from build123d import *

# Parameters (mm, degrees)
F1_DEPTH = 25
F2_R     = 1.2
F3_T     = -2.5
F4_DEPTH = 25
F6_DEPTH = 3
F7_SIZE  = 1.2


with BuildPart() as f1:
    # F0 (on Top) → F1 (new body)
    with BuildSketch(Plane.XY):
        with BuildLine():
            Line((0, -23.9775525033), (0, 0))
            Line((0, 0), (0, 26.0224474967))
            add(Edge.make_bspline(
                [(0, 26.0224474967), (-17.6971325381, 20.4363816506), (-33.2169395037, 16.3747998881), (-39.9791178567, 18.1051199008)],
                knots=[0, 0, 0, 0, 0.723504363, 0.723504363, 0.723504363, 0.723504363], degree=3))
            ThreePointArc((-39.9791178567, 18.1051199008), (-45.2661850168, 7.6441593667), (-56.9807893445, 7.2532375123))
            Line((-56.9807893445, 7.2532375123), (0, -23.9775525033))
        make_face()
        with BuildLine():
            ThreePointArc((-56.9807893445, 7.2532375123), (-45.2661850168, 7.6441593667), (-39.9791178567, 18.1051199008))
            Line((-39.9791178567, 18.1051199008), (-42.9724328811, 17.9049570556))
            ThreePointArc((-42.9724328811, 17.9049570556), (-54.0664587009, 9.2494171829), (-57.9998429251, 22.7595714353))
            Line((-57.9998429251, 22.7595714353), (-60.310319681, 24.6731275909))
            ThreePointArc((-60.310319681, 24.6731275909), (-62.749017961, 15.17887186), (-56.9807893445, 7.2532375123))
        make_face()
    extrude(amount=F1_DEPTH)

    # F2
    f2_edges = [f1.edges().sort_by_distance(p)[0] for p in [
        (-57.999843, 22.759571, 12.5),
        (-60.31032, 24.673128, 12.5),
        (-42.972433, 17.904957, 12.5),
    ]]
    fillet(f2_edges, radius=F2_R)

    # F3
    f3_openings = [f1.faces().sort_by_distance(p)[0] for p in [
        (-21.146453, 4.166771, 25),
    ]]
    offset(amount=F3_T, openings=f3_openings)

    # F4 (cut): a face of the model
    f4_faces = [f1.faces().sort_by_distance(p)[0] for p in [
        (-19.3393150943, 3.8306877566, 2.5),
    ]]
    extrude(f4_faces, amount=-F4_DEPTH, mode=Mode.SUBTRACT)

    # F5 (on face) → F6 (cut)
    with BuildSketch(Plane.YZ):
        with BuildLine():
            ThreePointArc((12.9166145043, 10), (13.5683701333, 11.1752351146), (13.7941155051, 12.5))
            ThreePointArc((13.7941155051, 12.5), (13.5683701333, 13.8247648854), (12.9166145043, 15))
            ThreePointArc((12.9166145043, 15), (5.7941155051, 12.5), (12.9166145043, 10))
        make_face()
        with BuildLine():
            ThreePointArc((20.5641841143, 12.5), (19.8319510673, 14.267766953), (18.0641841143, 15))
            ThreePointArc((18.0641841143, 15), (15.5641841143, 12.5), (18.0641841143, 10))
            ThreePointArc((18.0641841143, 10), (19.8319510673, 10.732233047), (20.5641841143, 12.5))
        make_face()
        with BuildLine():
            ThreePointArc((12.9166145043, 15), (13.5683701333, 13.8247648854), (13.7941155051, 12.5))
            ThreePointArc((13.7941155051, 12.5), (13.5683701333, 11.1752351146), (12.9166145043, 10))
            Line((12.9166145043, 10), (18.0641841143, 10))
            ThreePointArc((18.0641841143, 10), (15.5641841143, 12.5), (18.0641841143, 15))
            Line((18.0641841143, 15), (12.9166145043, 15))
        make_face()
    extrude(amount=-F6_DEPTH, mode=Mode.SUBTRACT)

    # F7
    f7_edges = [f1.edges().sort_by_distance(p)[0] for p in [
        (-2.5, 15.490399, 10),
        (-2.5, 15.490399, 15),
        (-2.5, 20.564184, 12.5),
    ]]
    chamfer(f7_edges, length=F7_SIZE)


solid = f1.part
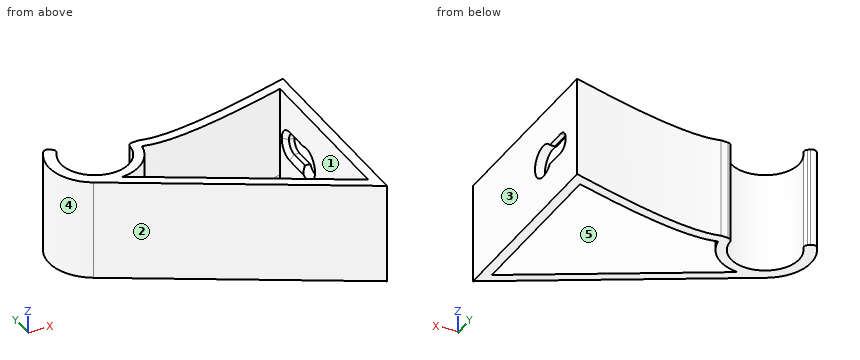
Part model, mm, in its own coordinate system. Face numbers are marked on the shaded views. A direction names the side the tool comes from. Round coordinates to 2 decimals unless told otherwise and drop trailing zeros. Write each loop counter-clockwise with the first axis right and the second up, starting at its lowest first coordinate (ties: lowest second). Pieces come first, ordered by that corner, then holes. Notation, with made-up numbers: M -24,48 L 1,48 A20 ccw 1,52 Z; hole C 79,35 d7. An arc over 180 degrees is marked long. Return JSON: item names as keys, results as strings. Group by question number.
(1) Drill centre lines: probe 1 along X at (y, z) = (13, 2.75); probe 2 along X at (y, z) = (14.5, 6); probe 3 along Y at (x, z) = (-42.5, 15). Where is each one in solid material? Low to high.
(2) Saw through at B-B on y = -3. Write the cut outline in (x, z).
(3) Saw through at C-C on x = -53. Write the cut outline in (y, z), then the cut area to 3 significant figures.
(4) Which spindle directions (+Z, -Z, +X, -X, +Y, -Y) get a long thin tool onto all of the face, cutting with end or side? Do the marked faces 1 and 2. Say none if no direction does.
(5) Pin check, flat tips, straight feed: pin 1 Ø5 at (y, z) = (-16.5, 12) entering from -X; pin 2 Ø3 at (x, z) = (-42, 7.5) entering from +Y; pin 3 Ø3 at (y, z) = (13, 12) entering from -X; pin 4 Ø10 at (x, y) = (-38.5, -12.5) entering from +Z. Stop position of each tip, or through.
(6) Saw through at A-A on x = -45.5. Write the cut outline in (y, z), then the cut area to 3 significant figures.
(7) Two-plate mould, pull along Y, no slides. Class the marked faces 3, 4 and 5: +Y half, -Y half, draft (parallel to the pull), parting line (faces both ways), or undercut.
Returned:
{
 "1": {"probe 1": "-62.1 to -58.76, -44.14 to -41.34, -2.5 to 0", "probe 2": "-62.6 to -59.47, -43.44 to -40.83, -2.5 to 0", "probe 3": "-0.68 to 2.17, 10.95 to 17.73"},
 "2": {"outline": "M -38.27,0 L -33.07,0 L -33.07,25 L -38.27,25 Z; M -2.5,0 L 0,0 L 0,25 L -2.5,25 Z"},
 "3": {"outline": "M 5.07,0 L 8.98,0 L 8.98,25 L 5.07,25 Z", "area": "97.7 mm²"},
 "4": {"face 1": "+Z, -Z", "face 2": "+Z, -Z, -X, -Y"},
 "5": {"pin 1": "x = -18.2", "pin 2": "y = 18.07", "pin 3": "x = -62.6", "pin 4": "through"},
 "6": {"outline": "M 0.96,0 L 3.81,0 L 3.81,25 L 0.96,25 Z; M 8.09,0 L 11.27,0 L 11.27,25 L 8.09,25 Z", "area": "151 mm²"},
 "7": {"face 3": "draft", "face 4": "parting line", "face 5": "undercut"}
}
